Input: dimensioned drawing with shaded views. Units: mm. Origin: part minimum x, y, z. Give positions to 0.01 mm unless a question says otherwise; leave off trailing zeros. Loops run counter-clockwise (first coordinate to the right, second up) from the corner with the lowest first, then second, coordinate; pieces in that order, holes last. Notation, with made-up numbers: M 30,-8 L 41,-8 A24 cw 41,24 Z; hole C 24,-10.75 d7. An arc over 180 degrees is marked long. Use CSV: the item, a comma, the result in double quotes. Start each with the question number.
Q1. Pin query (flat end, axial travel): pin 1 (6 mm diameter, centred on x = 3.5, z = 33, fed in from -Y); pin 2 (3 mm diameter, centred on x = 9, z = 21, fed in from -Y); pin 3 (1 mm diameter, centred on x = 7.5, z = 38, fed in from +Y); pin 4 (8 mm diameter, centred on y = 176, z = 23, fed in from +X). Return the tip coordinate at first contact, or that it passes through.
Q2. Section C-C, the plane y = 189.5. Output: boundary loops of the cut face in (x, z).
Q3. Section B-B, the plane x = 3. Output: boundary loops of the cut face in (y, z).
Q4. Pull-direction query (Y, two-part tool) for the marked faces 1, 2 and 3; classes: released by +Y, released by -Y, zero draft, split by the parting line, or undercut.
Q5. Material intervals for line 1 along Y through (x, z) = (4.25, 30); line 2 along Y through (x, z) = (2.75, 20); line 3 along Z through (x, y) = (4, 41), sorted ascending.
Q6. Section A-A, the plane z = 30. Output: boundary loops of the cut face in (x, y).
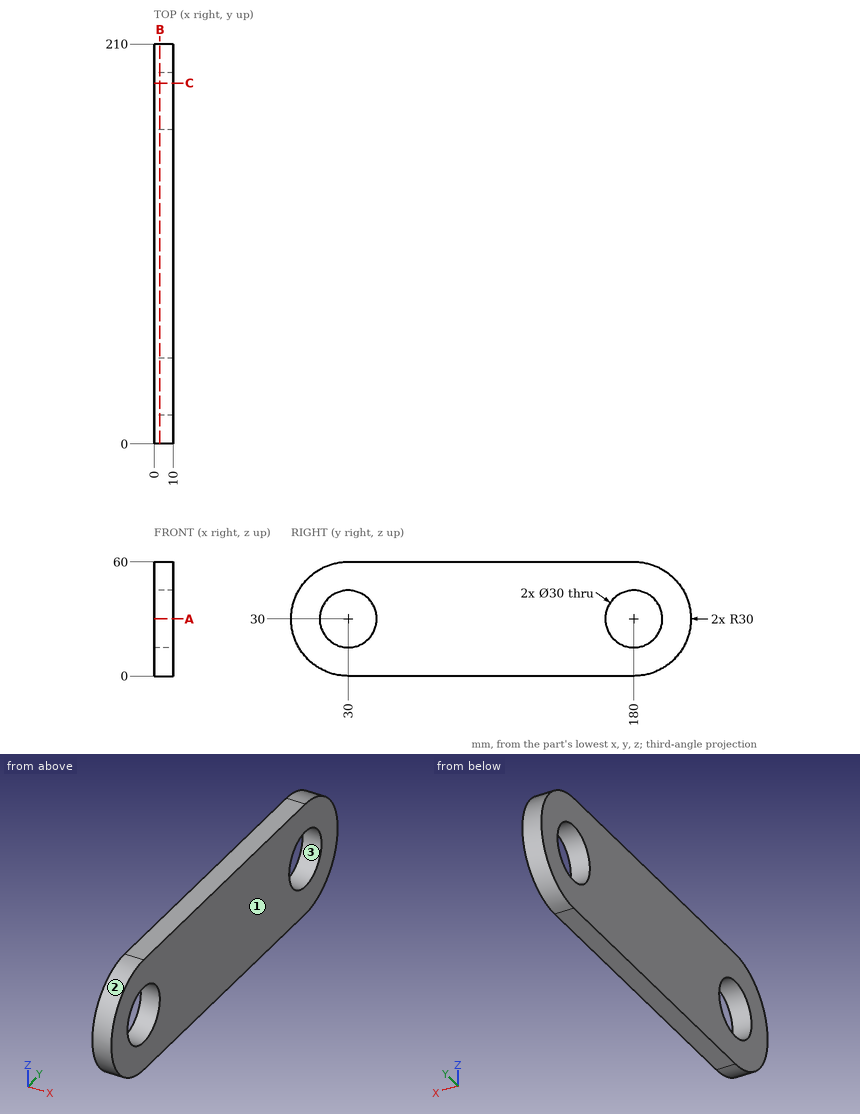
A:
1,pin 1,"y = 0"
1,pin 2,"y = 0.95"
1,pin 3,"y = 209.05"
1,pin 4,"through"
2,outline,"M 0,1.54 L 10,1.54 L 10,18.39 L 0,18.39 Z; M 0,41.61 L 10,41.61 L 10,58.46 L 0,58.46 Z"
3,outline,"M 30,0 L 180,0 A30 ccw 180,60 L 30,60 A30 ccw Z; hole C 30,30 d30; hole C 180,30 d30"
4,face 1,"zero draft"
4,face 2,"released by -Y"
4,face 3,"undercut"
5,line 1,"0 to 15, 45 to 165, 195 to 210"
5,line 2,"1.72 to 18.82, 41.18 to 168.82, 191.18 to 208.28"
5,line 3,"0 to 19.8, 40.2 to 60"
6,outline,"M 0,0 L 10,0 L 10,15 L 0,15 Z; M 0,45 L 10,45 L 10,165 L 0,165 Z; M 0,195 L 10,195 L 10,210 L 0,210 Z"
